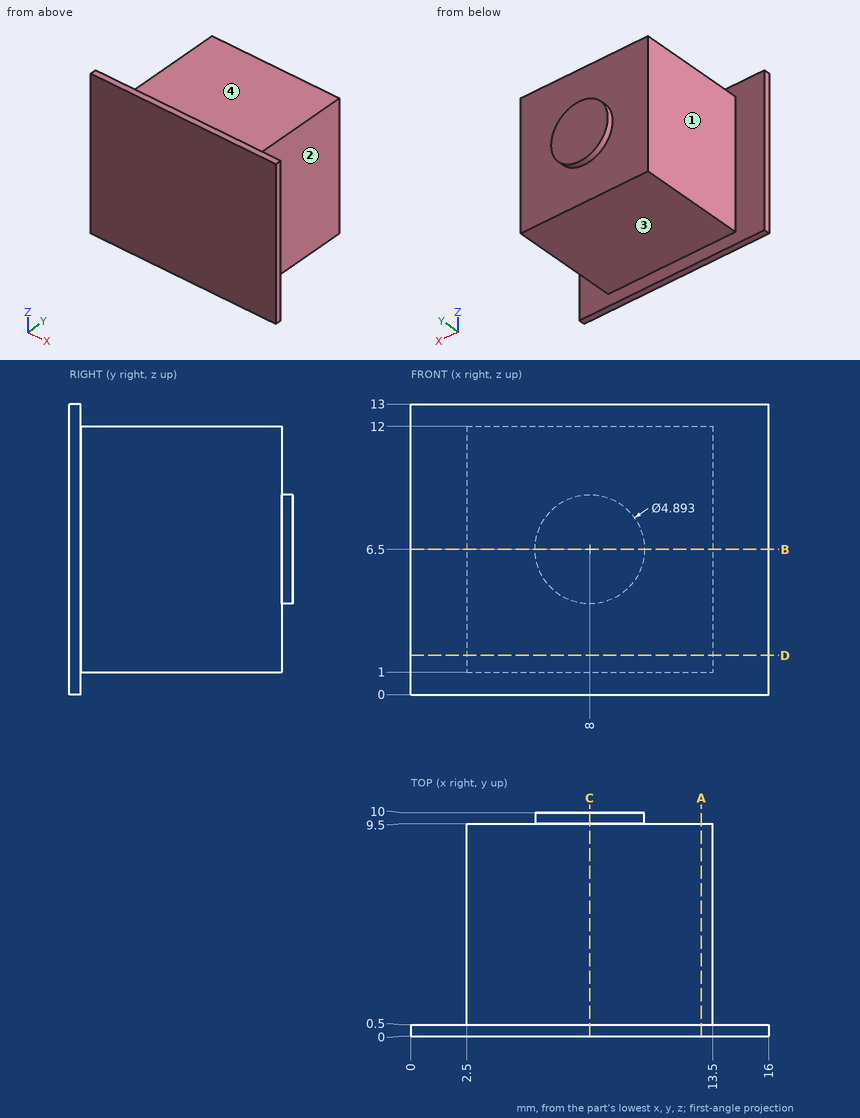
Can you work these out from the drawing? Everything is in mm from the part's minimum corner. A direction names the side the tool comes from. Round coordinates to 2 decimals unless told otherwise and drop trailing zeros. Order: outer loops, then holes, each group sorted by start corner. A loop starts at its lowest first (then second) coordinate and runs counter-clockwise, first axis right, second up. Notation, with made-up numbers: (14, 6.5) -> (70, 6.5) arc R27 cw to (70, 22.5) -> close; hole circle Ø6 at (21.5, 68.25). An arc over 180 degrees is marked (long way). Use CSV: the item, a comma, the result in double quotes.
1. Which directions (+Z, -Z, +X, -X, +Y, -Y) give clear straight access to the entire face, cutting with the end or side of a thin tool? Please do the marked faces 1, 2, 3 and 4.
Recorded:
face 1,"+Z, -Z, -X, +Y"
face 2,"+Z, -Z, +X, +Y"
face 3,"-Z, +X, -X, +Y"
face 4,"+Z, +X, -X, +Y"
2. I want a section at D-D on z = 1.75. List the corners of the cut face in (x, y) for me, and give its area (3 significant figures).
Recorded:
outline,"(0, 0) -> (16, 0) -> (16, 0.5) -> (13.5, 0.5) -> (13.5, 9.5) -> (2.5, 9.5) -> (2.5, 0.5) -> (0, 0.5) -> close"
area,"107 mm2"
3. I want a section at A-A on x = 13. List the corners of the cut face in (y, z) for me.
Recorded:
outline,"(0, 0) -> (0.5, 0) -> (0.5, 1) -> (9.5, 1) -> (9.5, 12) -> (0.5, 12) -> (0.5, 13) -> (0, 13) -> close"
4. I want a section at C-C on x = 8. List the corners of the cut face in (y, z) for me, and give its area (3 significant figures).
Recorded:
outline,"(0, 0) -> (0.5, 0) -> (0.5, 1) -> (9.5, 1) -> (9.5, 4.05) -> (10, 4.05) -> (10, 8.95) -> (9.5, 8.95) -> (9.5, 12) -> (0.5, 12) -> (0.5, 13) -> (0, 13) -> close"
area,"108 mm2"
5. I'm going to push flat-ended pins straight in: P1, Ø3, axis at x = 5, y = 7.5, coming from the -Z side; P2, Ø6, axis at y = 9, z = 4.5, coming from the -X side; P3, Ø1.5, axis at y = 4.5, z = 7, coming from the +X side. Where does each tip first touch, or does it pass through?
Recorded:
P1,"stops at z = 1"
P2,"stops at x = 2.5"
P3,"stops at x = 13.5"
6. I need wall thicknesses on line 1 along X through (y, z) = (9.25, 3.5); line 2 along Y through (x, z) = (1, 5); line 3 along Z through (x, y) = (4.5, 6.25). Which ranges of each line are inside material? Lowest first, please.
Recorded:
line 1,"x = 2.5 to 13.5"
line 2,"y = 0 to 0.5"
line 3,"z = 1 to 12"
7. I want a section at B-B on z = 6.5. List the corners of the cut face in (x, y) for me.
Recorded:
outline,"(0, 0) -> (16, 0) -> (16, 0.5) -> (13.5, 0.5) -> (13.5, 9.5) -> (10.45, 9.5) -> (10.45, 10) -> (5.55, 10) -> (5.55, 9.5) -> (2.5, 9.5) -> (2.5, 0.5) -> (0, 0.5) -> close"
